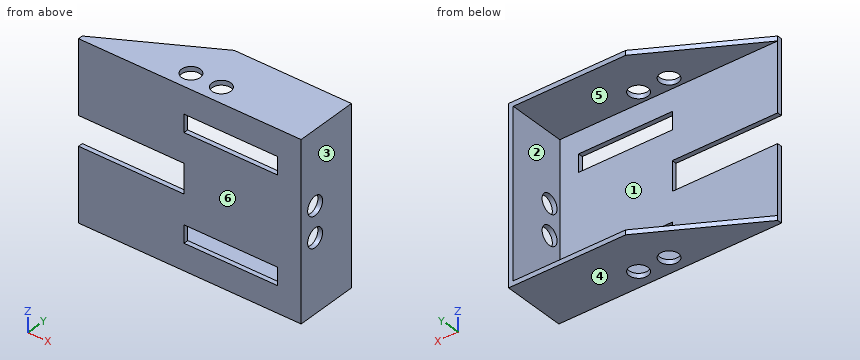
```python
from build123d import *

# Parameters (mm, degrees)
BOSS_EXTRUDE1_DEPTH = 4
BOSS_EXTRUDE2_DEPTH = 4
SKETCH3_W           = 142
SKETCH3_H           = 50
BOSS_EXTRUDE3_DEPTH = 4
SKETCH4_W           = 80
SKETCH4_H           = 15
CUT_EXTRUDE1_DEPTH  = 4
SKETCH5_R           = 8
CUT_EXTRUDE2_DEPTH  = 4
SKETCH6_R           = 8
CUT_EXTRUDE3_DEPTH  = 4


with BuildPart() as part:
    # Sketch1 → Boss-Extrude1 (new body)
    with BuildSketch(Plane(origin=(0, 0, 0), x_dir=(1, 0, 0), z_dir=(0, 1, 0))):
        Polygon((-5, -12.5), (-5, 12.5), (-95, 12.5), (-95, 75), (95, 75), (95, -75), (-95, -75), (-95, -12.5), align=None)
    extrude(amount=BOSS_EXTRUDE1_DEPTH)

    # Sketch2 → Boss-Extrude2 (add)
    with BuildSketch(Plane.XY.offset(75)):
        Polygon((95, 4), (95, 54), (-5, 54), (-95, 4), align=None)
    boss_extrude2 = extrude(amount=-BOSS_EXTRUDE2_DEPTH)

    # Mirror1: Boss-Extrude2 across plane
    add(boss_extrude2.mirror(Plane.XY))

    # Sketch3 → Boss-Extrude3 (add)
    with BuildSketch(Plane(origin=(95, 0, 0), x_dir=(0, 0, -1), z_dir=(1, 0, 0))):
        with Locations((0, 29)):
            Rectangle(SKETCH3_W, SKETCH3_H)
    extrude(amount=-BOSS_EXTRUDE3_DEPTH)

    # Sketch4 → Cut-Extrude1 (cut)
    with BuildSketch(Plane.XZ):
        with Locations((35, 45)):
            Rectangle(SKETCH4_W, SKETCH4_H)
    cut_extrude1 = extrude(amount=-CUT_EXTRUDE1_DEPTH, mode=Mode.SUBTRACT)

    # Mirror2: Cut-Extrude1 across plane
    add(cut_extrude1.mirror(Plane.XY), mode=Mode.SUBTRACT)

    # Sketch5 → Cut-Extrude2 (cut)
    with BuildSketch(Plane(origin=(95, 0, 0), x_dir=(0, 0, -1), z_dir=(1, 0, 0))):
        with Locations((-13, 15)):
            Circle(SKETCH5_R)
        with Locations((13, 15)):
            Circle(SKETCH5_R)
    extrude(amount=-CUT_EXTRUDE2_DEPTH, mode=Mode.SUBTRACT)

    # Sketch6 → Cut-Extrude3 (cut)
    with BuildSketch(Plane(origin=(0, 0, -75), x_dir=(-1, 0, 0), z_dir=(0, 0, -1))):
        with Locations((-15, 15)):
            Circle(SKETCH6_R)
        with Locations((11, 15)):
            Circle(SKETCH6_R)
    cut_extrude3 = extrude(amount=-CUT_EXTRUDE3_DEPTH, mode=Mode.SUBTRACT)

    # Mirror3: Cut-Extrude3 across plane
    add(cut_extrude3.mirror(Plane.XY), mode=Mode.SUBTRACT)


solid = part.part
```
Input: part model. Units: mm. Frame: model coordinates. Face numbers are marked on the shaded views. A direction names the side the tool comes from. Coordinates: 2 decimals unless noted, no trailing zeros. Loops run counter-clockwise (first coordinate to the right, second up) from the corner with the lowest first, then second, coordinate; pieces in that order, holes last. Notation, with made-up numbers: M -9,12.25 L 41,12.25 A24 cw 41,39.25 Z; hole C -23,2.5 d1. An arc over 180 degrees is marked long. Use a Markdown table: item, result. Add a question column.
1) Set-up query: the marked faces 5 and 6. Return all of +Z, -Z, +X, -X, +Y, -Y with unobstructed straight access to the full face (end or side cutting, diameter ignored); none if empty.
2) Section A-A, the plane y = 15. Give the number of separate pieces and of enclosed holes in the cut face, plus the area to 3 significant figures.
3) Pin query (flat end, axial travel): P1, Ø21, axis at x = -11, y = 15, coming from the -Z side; P2, Ø1.5, axis at y = 35.5, z = 52, coming from the -X side; P3, Ø3, axis at y = 2, z = 4, coming from the -X side; P4, Ø10, axis at x = 31, z = 49.5, coming from the +Y side. Return the tip coordinate at first contact, or that it passes through.
4) Draft query along Z for the marked faces 1, 2, 3 and 4. Return one class per face: +Z half, -Z half, draft (parallel to the pull), parting line (faces both ways), or undercut.
5) Section C-C, the plane z = -46.5. Return the cut outline in (x, y), plus the area to 3 significant figures.
6) Section B-B, the plane x = 15. Return the cut outline in (y, z).
7) Line query: L1, parallel to Y at x = 93.9, z = 13; L2, parallel to Z at x = -6.5, y = 5.5; L3, parallel to X at y = 18, z = 31. Output: solid intervals per line, ascending. Write a range as from..to.
8) Section D-D, the plane x = -8. Return the cut outline in (y, z).
Answer below:
| question | item | result |
|---|---|---|
| 1 | face 5 | -X, +Y |
| 1 | face 6 | +Z, -Z, +X, -X, -Y |
| 2 | separate pieces | 7 |
| 2 | enclosed holes | 0 |
| 2 | area | 1,550 mm2 |
| 3 | P1 | z = -75 |
| 3 | P2 | x = 91 |
| 3 | P3 | x = -5 |
| 3 | P4 | y = 4 |
| 4 | face 1 | undercut |
| 4 | face 2 | undercut |
| 4 | face 3 | draft |
| 4 | face 4 | -Z half |
| 5 | outline | M -95,0 L -5,0 L -5,4 L -95,4 Z; M 75,0 L 95,0 L 95,54 L 91,54 L 91,4 L 75,4 Z |
| 5 | area | 640 mm2 |
| 6 | outline | M 0,-75 L 7,-75 L 7,-71 L 4,-71 L 4,-52.5 L 0,-52.5 Z; M 0,-37.5 L 4,-37.5 L 4,37.5 L 0,37.5 Z; M 0,52.5 L 4,52.5 L 4,71 L 7,71 L 7,75 L 0,75 Z; M 23,-75 L 54,-75 L 54,-71 L 23,-71 Z; M 23,71 L 54,71 L 54,75 L 23,75 Z |
| 7 | L1 | 0..7, 23..54 |
| 7 | L2 | -75..-71, 71..75 |
| 7 | L3 | 91..95 |
| 8 | outline | M 0,-75 L 7.58,-75 L 7.58,-71 L 4,-71 L 4,-12.5 L 0,-12.5 Z; M 0,12.5 L 4,12.5 L 4,71 L 7.58,71 L 7.58,75 L 0,75 Z; M 22.42,-75 L 52.33,-75 L 52.33,-71 L 22.42,-71 Z; M 22.42,71 L 52.33,71 L 52.33,75 L 22.42,75 Z |
